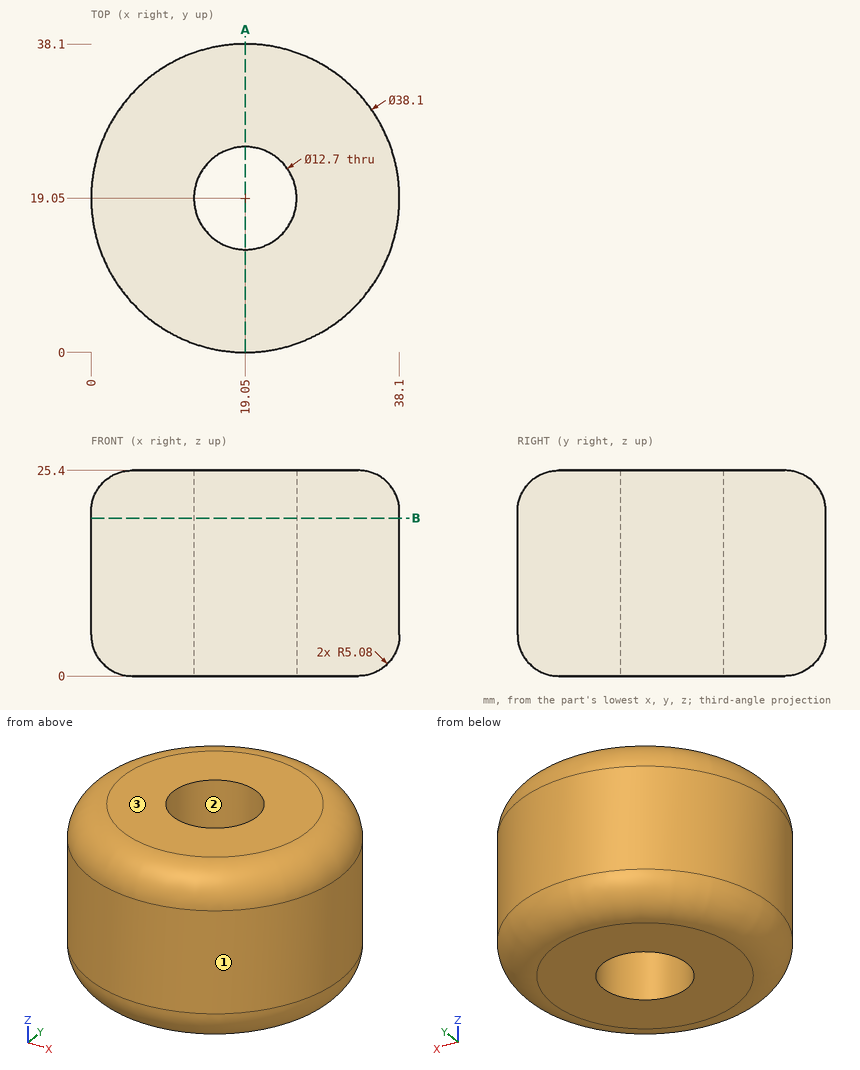
Here's the drawing with two shaded views (mm, measured from the low corner). I have some questions. Give positions to 0.01 mm unless a question says otherwise; leave off trailing zeros. Order: outer loops, then holes, each group sorted by start corner. A loop starts at its lowest first (then second) coordinate and runs counter-clockwise, first axis right, second up. Notation, with made-up numbers: (80.5, 70.25) - (118.5, 70.25) arc R15 cw to (118.5, 90.25) - close; hole circle Ø1 at (6.5, 17). An arc over 180 degrees is marked (long way). Write each question's results on one line, items separated by ' | '.
1) Suppose I cut it at B-B, the plane z = 19.5. Write out the boundary of the cut face in (x, y).
Final values:
outline: circle Ø38.1 at (19.05, 19.05); hole circle Ø12.7 at (19.05, 19.05)
2) Please list where these lines run through material, in increasing order: line 1 along Y through (x, z) = (19.05, 15); line 2 along Y through (x, z) = (15, 15); line 3 along X through (y, z) = (20.5, 19.25). Write a range as [from, to].
Final values:
line 1: y = [0, 12.7], [25.4, 38.1] | line 2: y = [0.44, 14.16], [23.94, 37.66] | line 3: x = [0.06, 12.87], [25.23, 38.04]
3) If we mould it in two halves opening along Y, with no side actions, what happens to the marked faces 1, 2 and 3? For each: pulls with the +Y half, pulls with the -Y half, needs draft (parallel to the pull), parting line crosses it, or undercut.
Final values:
face 1: parting line crosses it | face 2: undercut | face 3: needs draft
4) Suppose I cut it at A-A, the plane x = 19.05. Write out the boundary of the cut face in (y, z), then the cut area to 3 significant figures.
Final values:
outline: (0, 5.08) arc R5.08 ccw to (5.08, 0) - (12.7, 0) - (12.7, 25.4) - (5.08, 25.4) arc R5.08 ccw to (0, 20.32) - close; (25.4, 0) - (33.02, 0) arc R5.08 ccw to (38.1, 5.08) - (38.1, 20.32) arc R5.08 ccw to (33.02, 25.4) - (25.4, 25.4) - close | area: 623 mm^2
5) I'm going to push flat-ended pins straight in: pin 1 Ø5 at (x, z) = (29.5, 19) entering from +Y; pin 2 Ø3 at (x, z) = (21.5, 15.5) entering from -Y; pin 3 Ø8 at (x, z) = (12.5, 12) entering from -Y. Where does each tip first touch, or does it pass through?
Final values:
pin 1: stops at y = 36.36 | pin 2: stops at y = 0.02 | pin 3: stops at y = 0.17
